Part model, mm, in its own coordinate system. A direction names the side the tool comes from. Round coordinates to 2 decimals unless told otherwise and drop trailing zeros. Loops run counter-clockwise (first coordinate to the right, second up) from the corner with the lowest first, then second, coordinate; pieces in that order, holes last. Notation, with made-up numbers: M 42,38 L 76,38 A21 cw 76,59 Z; hole C 88,-22.75 d8. An arc over 180 degrees is marked long. Write each question's results on one line, items separated by ' | '.
from build123d import *

# Parameters (mm, degrees)
SKETCH1_R           = 3.175
BOSS_EXTRUDE1_DEPTH = 6.35
SKETCH10_W          = 19.685
SKETCH10_H          = 81.28
SKETCH10_R          = 3.175
BOSS_EXTRUDE4_DEPTH = 17.78
SKETCH12_W          = 17.145
SKETCH12_H          = 81.28
CUT_EXTRUDE5_DEPTH  = 12.7
SKETCH14_R          = 6.35
CUT_EXTRUDE9_DEPTH  = 1.27
CHAMFER2_SIZE       = 0.635
SKETCH15_W          = 63.5
SKETCH15_H          = 12.7
CUT_EXTRUDE10_DEPTH = 36.576
SKETCH16_W          = 17.145
SKETCH16_H          = 6.35
CUT_EXTRUDE11_DEPTH = 84.836
FILLET1_R           = 1.27
FILLET2_START       = -31.75
FILLET2_DEPTH       = 6.3500001
FILLET2_START_2     = 25.3999999
FILLET2_2_DEPTH     = 6.3500001
FILLET2_START_3     = -30
FILLET2_3_DEPTH     = 6.505


with BuildPart() as part:
    # Sketch1 → Boss-Extrude1 (new body)
    with BuildSketch(Plane(origin=(0, 0, 0), x_dir=(1, 0, 0), z_dir=(0, 1, 0))):
        Polygon((0, 40.64), (38.1, 13.962092794), (38.1, -13.962092794), (0, -40.64), (-44.45, -40.64), (-44.45, 40.64), align=None)
        with Locations(Location((-36.83, 33.02, 0), (0, 0, 270))):
            Circle(SKETCH1_R, mode=Mode.SUBTRACT)
        with Locations(Location((-36.83, -33.02, 0), (0, 0, 270))):
            Circle(SKETCH1_R, mode=Mode.SUBTRACT)
        with BuildLine():
            Line((-5.08, 19.05), (5.08, 19.05))
            ThreePointArc((5.08, 19.05), (8.255, 15.875), (5.08, 12.7))
            Line((5.08, 12.7), (-5.08, 12.7))
            ThreePointArc((-5.08, 12.7), (-8.255, 15.875), (-5.08, 19.05))
        make_face(mode=Mode.SUBTRACT)
        with BuildLine():
            Line((-5.08, -12.7), (5.08, -12.7))
            ThreePointArc((5.08, -12.7), (8.255, -15.875), (5.08, -19.05))
            Line((5.08, -19.05), (-5.08, -19.05))
            ThreePointArc((-5.08, -19.05), (-8.255, -15.875), (-5.08, -12.7))
        make_face(mode=Mode.SUBTRACT)
        with BuildLine():
            Line((22.41630657, 3.175), (32.57630657, 3.175))
            ThreePointArc((32.57630657, 3.175), (35.75130657, 0), (32.57630657, -3.175))
            Line((32.57630657, -3.175), (22.41630657, -3.175))
            ThreePointArc((22.41630657, -3.175), (19.24130657, 0), (22.41630657, 3.175))
        make_face(mode=Mode.SUBTRACT)
    extrude(amount=BOSS_EXTRUDE1_DEPTH)

    # Sketch10 → Boss-Extrude4 (add)
    with BuildSketch(Plane(origin=(0, 6.35, 0), x_dir=(1, 0, 0), z_dir=(0, 1, 0))):
        with Locations((-34.6075, 0)):
            Rectangle(SKETCH10_W, SKETCH10_H)
        with Locations(Location((-36.83, -33.02, 0), (0, 0, 270))):
            Circle(SKETCH10_R, mode=Mode.SUBTRACT)
        with Locations(Location((-36.83, 33.02, 0), (0, 0, 270))):
            Circle(SKETCH10_R, mode=Mode.SUBTRACT)
    extrude(amount=BOSS_EXTRUDE4_DEPTH)

    # Sketch12 → Cut-Extrude5 (cut)
    with BuildSketch(Plane.XZ):
        with Locations((-35.8775, 0)):
            Rectangle(SKETCH12_W, SKETCH12_H)
    extrude(amount=-CUT_EXTRUDE5_DEPTH, mode=Mode.SUBTRACT)

    # Sketch14 → Cut-Extrude9 (cut)
    with BuildSketch(Plane(origin=(0, 24.13, 0), x_dir=(1, 0, 0), z_dir=(0, 1, 0))):
        with Locations(Location((-36.83, 33.02, 0), (0, 0, 270))):
            Circle(SKETCH14_R)
        with Locations(Location((-36.83, -33.02, 0), (0, 0, 270))):
            Circle(SKETCH14_R)
    extrude(amount=-CUT_EXTRUDE9_DEPTH, mode=Mode.SUBTRACT)

    # Chamfer2
    chamfer2_edges = [part.edges().sort_by_distance(p)[0] for p in [
        (-36.83, 22.86, -36.195),
        (-36.83, 22.86, 29.845),
    ]]
    chamfer(chamfer2_edges, length=CHAMFER2_SIZE)

    # Sketch15 → Cut-Extrude10 (cut)
    with BuildSketch(Plane(origin=(-24.765, 0, 0), x_dir=(0, 0, -1), z_dir=(1, 0, 0))):
        with Locations((0, 12.7)):
            Rectangle(SKETCH15_W, SKETCH15_H)
    extrude(amount=-CUT_EXTRUDE10_DEPTH, mode=Mode.SUBTRACT)

    # Sketch16 → Cut-Extrude11 (cut)
    with BuildSketch(Plane(origin=(0, 0, -40.64), x_dir=(-1, 0, 0), z_dir=(0, 0, -1))):
        with Locations((35.8775, 15.875)):
            Rectangle(SKETCH16_W, SKETCH16_H)
    extrude(amount=-CUT_EXTRUDE11_DEPTH, mode=Mode.SUBTRACT)

    # Fillet1
    fillet1_edges = [part.edges().sort_by_distance(p)[0] for p in [
        (-24.765, 6.35, -36.195),
        (-27.305, 19.05, 36.195),
        (-27.305, 19.05, -36.195),
        (-24.765, 6.35, 36.195),
    ]]
    fillet(fillet1_edges, radius=FILLET1_R)

    # Fillet2: read off the stored shape, not the designer's step
    # Fillet2 outline → Fillet2 (add)
    with BuildSketch(Plane.XY.offset(FILLET2_START)):
        with BuildLine():
            ThreePointArc((-23.495, 6.35), (-24.393025612, 6.721974388), (-24.765, 7.62))
            Line((-24.765, 7.62), (-24.765, 19.05))
            Line((-24.765, 19.05), (-28.575, 19.05))
            ThreePointArc((-28.575, 19.05), (-27.676974388, 18.678025612), (-27.305, 17.78))
            Line((-27.305, 17.78), (-27.305, 6.35))
            Line((-27.305, 6.35), (-23.495, 6.35))
        make_face()
    extrude(amount=FILLET2_DEPTH)

    # Fillet2 2 outline → Fillet2 2 (add)
    with BuildSketch(Plane.XY.offset(FILLET2_START_2)):
        with BuildLine():
            ThreePointArc((-23.495, 6.35), (-24.393025612, 6.721974388), (-24.765, 7.62))
            Line((-24.765, 7.62), (-24.765, 19.05))
            Line((-24.765, 19.05), (-28.575, 19.05))
            ThreePointArc((-28.575, 19.05), (-27.676974388, 18.678025612), (-27.305, 17.78))
            Line((-27.305, 17.78), (-27.305, 6.35))
            Line((-27.305, 6.35), (-23.495, 6.35))
        make_face()
    extrude(amount=FILLET2_2_DEPTH)

    # Fillet2 3 outline → Fillet2 3 (cut)
    with BuildSketch(Plane.YZ.offset(FILLET2_START_3)):
        with BuildLine():
            ThreePointArc((19.05, 25.4), (17.190128061, 29.890128061), (12.7, 31.75))
            ThreePointArc((12.7, 31.75), (8.209871939, 29.890128061), (6.35, 25.4))
            Line((6.35, 25.4), (19.05, 25.4))
        make_face()
        with BuildLine():
            ThreePointArc((12.7, -31.75), (17.190128061, -29.890128061), (19.05, -25.4))
            Line((19.05, -25.4), (6.35, -25.4))
            ThreePointArc((6.35, -25.4), (8.209871939, -29.890128061), (12.7, -31.75))
        make_face()
    extrude(amount=FILLET2_3_DEPTH, mode=Mode.SUBTRACT)

    # Chamfer3: read off the stored shape, not the designer's step
    # Chamfer3: loft between two sections, ruled curve by curve
    chamfer3_from = [
        Edge.make_three_point_arc((-5.08, 3.81, 12.7), (-7.32506403, 3.81, 13.62993597), (-8.255, 3.81, 15.875)),
        Edge.make_three_point_arc((-8.255, 3.81, 15.875), (-7.32506403, 3.81, 18.12006403), (-5.08, 3.81, 19.05)),
        Edge.make_three_point_arc((5.08, 3.81, 19.05), (7.32506403, 3.81, 18.12006403), (8.255, 3.81, 15.875)),
        Edge.make_three_point_arc((8.255, 3.81, 15.875), (7.32506403, 3.81, 13.62993597), (5.08, 3.81, 12.7)),
        Edge.make_line((5.08, 3.81, 12.7), (-5.08, 3.81, 12.7)),
        Edge.make_line((-5.08, 3.81, 19.05), (5.08, 3.81, 19.05)),
    ]
    chamfer3_to = [
        Edge.make_three_point_arc((-5.08, 6.35, 10.16), (-9.121115254, 6.35, 11.833884746), (-10.795, 6.35, 15.875)),
        Edge.make_three_point_arc((-10.795, 6.35, 15.875), (-9.121115254, 6.35, 19.916115254), (-5.08, 6.35, 21.59)),
        Edge.make_three_point_arc((5.08, 6.35, 21.59), (9.121115254, 6.35, 19.916115254), (10.795, 6.35, 15.875)),
        Edge.make_three_point_arc((10.795, 6.35, 15.875), (9.121115254, 6.35, 11.833884746), (5.08, 6.35, 10.16)),
        Edge.make_line((5.08, 6.35, 10.16), (-5.08, 6.35, 10.16)),
        Edge.make_line((-5.08, 6.35, 21.59), (5.08, 6.35, 21.59)),
    ]
    chamfer3 = Solid(Shell([*[Face.make_surface_from_curves(chamfer3_from[k], chamfer3_to[k]) for k in range(6)], Face(Wire(chamfer3_from)), Face(Wire(chamfer3_to))]))
    add(chamfer3, mode=Mode.SUBTRACT)

    # Chamfer3 2: loft between two sections, ruled curve by curve
    chamfer3_2_from = [
        Edge.make_three_point_arc((22.41630657, 3.81, -3.175), (20.17124254, 3.81, -2.24506403), (19.24130657, 3.81, 0)),
        Edge.make_three_point_arc((19.24130657, 3.81, 0), (20.17124254, 3.81, 2.24506403), (22.41630657, 3.81, 3.175)),
        Edge.make_three_point_arc((32.57630657, 3.81, 3.175), (34.8213706, 3.81, 2.24506403), (35.75130657, 3.81, 0)),
        Edge.make_three_point_arc((35.75130657, 3.81, 0), (34.8213706, 3.81, -2.24506403), (32.57630657, 3.81, -3.175)),
        Edge.make_line((32.57630657, 3.81, -3.175), (22.41630657, 3.81, -3.175)),
        Edge.make_line((22.41630657, 3.81, 3.175), (32.57630657, 3.81, 3.175)),
    ]
    chamfer3_2_to = [
        Edge.make_three_point_arc((22.41630657, 6.35, -5.715), (18.375191316, 6.35, -4.041115254), (16.70130657, 6.35, 0)),
        Edge.make_three_point_arc((16.70130657, 6.35, 0), (18.375191316, 6.35, 4.041115254), (22.41630657, 6.35, 5.715)),
        Edge.make_three_point_arc((32.57630657, 6.35, 5.715), (36.617421825, 6.35, 4.041115254), (38.29130657, 6.35, 0)),
        Edge.make_three_point_arc((38.29130657, 6.35, 0), (36.617421825, 6.35, -4.041115254), (32.57630657, 6.35, -5.715)),
        Edge.make_line((32.57630657, 6.35, -5.715), (22.41630657, 6.35, -5.715)),
        Edge.make_line((22.41630657, 6.35, 5.715), (32.57630657, 6.35, 5.715)),
    ]
    chamfer3_2 = Solid(Shell([*[Face.make_surface_from_curves(chamfer3_2_from[k], chamfer3_2_to[k]) for k in range(6)], Face(Wire(chamfer3_2_from)), Face(Wire(chamfer3_2_to))]))
    add(chamfer3_2, mode=Mode.SUBTRACT)

    # Chamfer3 3: loft between two sections, ruled curve by curve
    chamfer3_3_from = [
        Edge.make_three_point_arc((-5.08, 3.81, -19.05), (-7.32506403, 3.81, -18.12006403), (-8.255, 3.81, -15.875)),
        Edge.make_three_point_arc((-8.255, 3.81, -15.875), (-7.32506403, 3.81, -13.62993597), (-5.08, 3.81, -12.7)),
        Edge.make_three_point_arc((5.08, 3.81, -12.7), (7.32506403, 3.81, -13.62993597), (8.255, 3.81, -15.875)),
        Edge.make_three_point_arc((8.255, 3.81, -15.875), (7.32506403, 3.81, -18.12006403), (5.08, 3.81, -19.05)),
        Edge.make_line((5.08, 3.81, -19.05), (-5.08, 3.81, -19.05)),
        Edge.make_line((-5.08, 3.81, -12.7), (5.08, 3.81, -12.7)),
    ]
    chamfer3_3_to = [
        Edge.make_three_point_arc((-5.08, 6.35, -21.59), (-9.121115254, 6.35, -19.916115254), (-10.795, 6.35, -15.875)),
        Edge.make_three_point_arc((-10.795, 6.35, -15.875), (-9.121115254, 6.35, -11.833884746), (-5.08, 6.35, -10.16)),
        Edge.make_three_point_arc((5.08, 6.35, -10.16), (9.121115254, 6.35, -11.833884746), (10.795, 6.35, -15.875)),
        Edge.make_three_point_arc((10.795, 6.35, -15.875), (9.121115254, 6.35, -19.916115254), (5.08, 6.35, -21.59)),
        Edge.make_line((5.08, 6.35, -21.59), (-5.08, 6.35, -21.59)),
        Edge.make_line((-5.08, 6.35, -10.16), (5.08, 6.35, -10.16)),
    ]
    chamfer3_3 = Solid(Shell([*[Face.make_surface_from_curves(chamfer3_3_from[k], chamfer3_3_to[k]) for k in range(6)], Face(Wire(chamfer3_3_from)), Face(Wire(chamfer3_3_to))]))
    add(chamfer3_3, mode=Mode.SUBTRACT)


solid = part.part
Item 1: Band-saw the part on D-D on y = 20.25. Give the cut face in (x, z) (3 decimals).
Filled sheet:
outline: M -44.45,-40.64 L -24.765,-40.64 L -24.765,40.64 L -44.45,40.64 Z; hole C -36.83,-33.02 d6.35; hole C -36.83,33.02 d6.35
Item 2: Drop flat-ended pins along their axis: P1, Ø2, axis at x = -1.5, z = -27, coming from the +Y side; P2, Ø10, axis at x = -34, z = 12, coming from the -Y side; P3, Ø10, axis at x = 15.5, y = 3, coming from the -Z side; P4, Ø5, axis at x = -36.83, z = 33.02, coming from the +Y side. Give the stop position or say it passes through.
Filled sheet:
P1: y = 6.35 | P2: y = 19.05 | P3: z = -33.29 | P4: through
Item 3: Band-saw the part on B-B on z = -33.02. Give the cut face in (x, y) (3 decimals), and give its area (3 significant figures).
Filled sheet:
outline: M -44.45,19.05 L -40.005,19.05 L -40.005,22.225 L -40.64,22.86 L -43.18,22.86 L -43.18,24.13 L -44.45,24.13 Z; M -33.655,19.05 L -28.575,19.05 A1.27 cw -27.305,17.78 L -27.305,0 L 10.882,0 L 10.882,6.35 L -23.495,6.35 A1.27 cw -24.765,7.62 L -24.765,24.13 L -30.48,24.13 L -30.48,22.86 L -33.02,22.86 L -33.655,22.225 Z | area: 335 mm^2
Item 4: Wall check: L1, parallel to Z at x = -36.83, y = 19.95 (3 decimals); L2, parallel to X at y = 21.4, z = -33.02 (3 decimals); L3, parallel to X at y = 23.2, z = 33.02 (3 decimals). Give the ranges that are in metal, low to high.
Filled sheet:
L1: -40.64 to -36.195, -29.845 to 29.845, 36.195 to 40.64 | L2: -44.45 to -40.005, -33.655 to -24.765 | L3: -44.45 to -43.18, -30.48 to -24.765
Item 5: Which spindle directions (+Z, -Z, +X, -X, +Y, -Y) get a long thin tool onto all of the face, cutting with end or side? Do faces 5 (the cylindrical face through (19.242, 1.878, 0.07)), 6 (the flat face through (-40, 22.86, 36)), 7 (the flat face through (-1, 0, -1)). Say none if no direction does.
Filled sheet:
face 5: +Y, -Y | face 6: +Y | face 7: +Z, -Z, +X, -X, -Y
Item 6: Two-plate mould, pull along Z, no slides. Class faces 1 (the flat face through (38.1, 3, 0)), 2 (the flat face through (19.32, 3.13, 27.11)), 3 (the flat face through (18.78, 3.13, -27.49)), 4 (the flat face through (0, 2, -12.7)): +Z half, -Z half, draft (parallel to the pull), parting line (faces both ways), or undercut.
Filled sheet:
face 1: draft | face 2: +Z half | face 3: -Z half | face 4: undercut
Item 7: Band-saw the part on A-A on x = -36.83. Give the cut face in (y, z) (3 decimals), and give its area (3 significant figures).
Filled sheet:
outline: M 19.05,-40.64 L 24.13,-40.64 L 24.13,-39.37 L 22.86,-39.37 L 22.86,-36.83 L 22.225,-36.195 L 19.05,-36.195 Z; M 19.05,-29.845 L 22.225,-29.845 L 22.86,-29.21 L 22.86,-26.67 L 24.13,-26.67 L 24.13,26.67 L 22.86,26.67 L 22.86,29.21 L 22.225,29.845 L 19.05,29.845 Z; M 19.05,36.195 L 22.225,36.195 L 22.86,36.83 L 22.86,39.37 L 24.13,39.37 L 24.13,40.64 L 19.05,40.64 Z | area: 331 mm^2
Item 8: Band-saw the part on C-C on y = 11.75. Give the cut face in (x, z) (3 decimals), and give its area (3 significant figures).
Filled sheet:
outline: M -27.305,-40.64 L -24.765,-40.64 L -24.765,-31.679 L -27.305,-31.679 Z; M -27.305,31.679 L -24.765,31.679 L -24.765,40.64 L -27.305,40.64 Z | area: 45.5 mm^2
